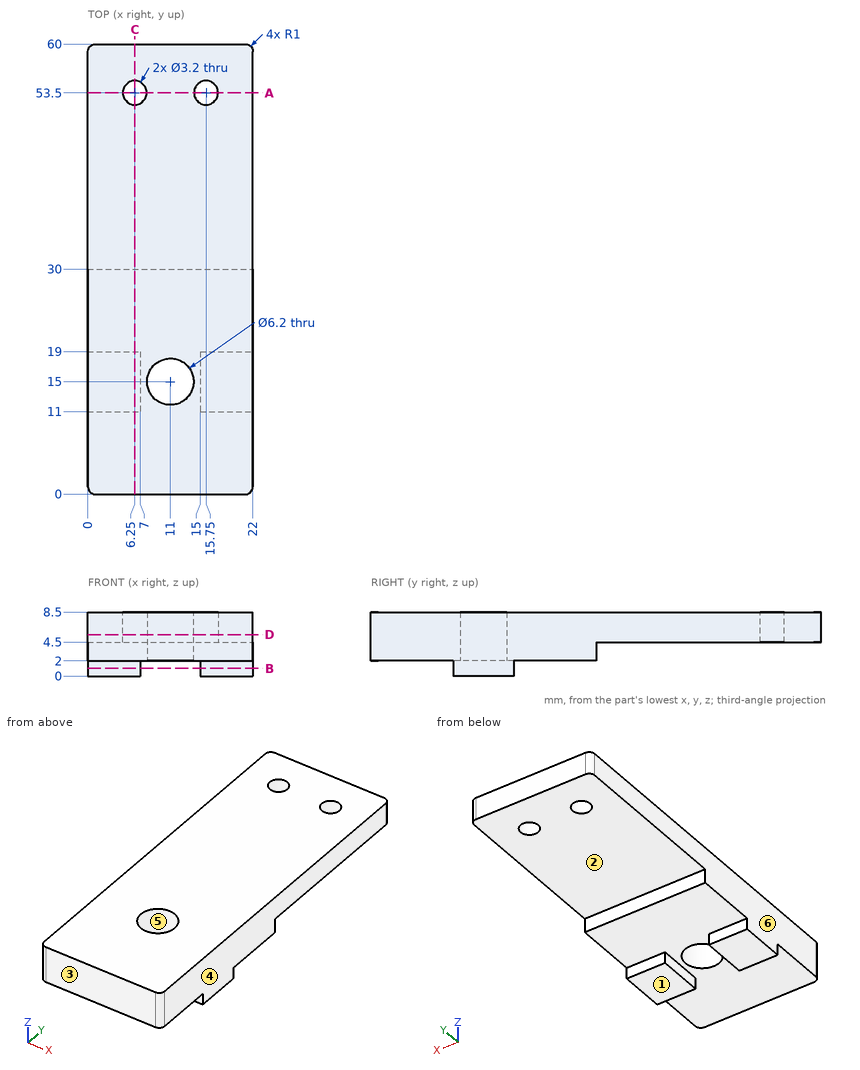
Source: three-view drawing plus pictorial views. Frame: mm from the lowest corner of the part. A direction names the side the tool comes from. Coordinates: 2 decimals unless noted, no trailing zeros. Write each loop counter-clockwise with the first axis right and the second up, starting at its lowest first coordinate (ties: lowest second). Pieces come first, ordered by that corner, then holes. Notation, with made-up numbers: (26, 61) -> (54, 61) arc R27 ccw to (54, 89) -> close; hole circle Ø11 at (62, 26). An arc over 180 degrees is marked (long way). Write each question's results on one line, items separated by ' | '.
Item 1: Set-up query: the marked faces 1 and 2. Return all of +Z, -Z, +X, -X, +Y, -Y with unobstructed straight access to the full face (end or side cutting, diameter ignored); none if empty.
Conclusion:
face 1: -Z, +X, -X, +Y, -Y | face 2: -Z, +X, -X, +Y
Item 2: Section query A-A on y = 53.5. Return loops of the section in (x, z).
Conclusion:
outline: (0, 4.5) -> (4.65, 4.5) -> (4.65, 8.5) -> (0, 8.5) -> close; (7.85, 4.5) -> (14.15, 4.5) -> (14.15, 8.5) -> (7.85, 8.5) -> close; (17.35, 4.5) -> (22, 4.5) -> (22, 8.5) -> (17.35, 8.5) -> close
Item 3: Pin query (flat end, axial travel): pin 1 Ø0.6 at (x, z) = (18, 1) entering from +Y; pin 2 Ø5 at (x, y) = (18, 40) entering from -Z; pin 3 Ø5 at (x, y) = (18, 25.5) entering from -Z; pin 4 Ø2.5 at (x, y) = (15.75, 53.5) entering from +Z. Return the tip coordinate at first contact, or that it passes through.
Conclusion:
pin 1: stops at y = 19 | pin 2: stops at z = 4.5 | pin 3: stops at z = 2 | pin 4: passes through
Item 4: Mould query, pull axis X, two halves, no side actions, for the marked faces 3, 4, 5 and 6. Classes: +X half, -X half, draft (parallel to the pull), parting line (faces both ways), or undercut.
Conclusion:
face 3: draft | face 4: +X half | face 5: undercut | face 6: -X half
Item 5: Material intervals for probe 1 along X at (y, z) = (15, 6.75); probe 2 along Y at (x, z) = (6.25, 5.95); probe 3 along Z at (x, y) = (18.75, 7), sorted ascending.
Conclusion:
probe 1: x = 0 to 7.9, 14.1 to 22 | probe 2: y = 0 to 51.9, 55.1 to 60 | probe 3: z = 2 to 8.5
Item 6: Section query B-B on z = 1. Return loops of the section in (x, y).
Conclusion:
outline: (0, 11) -> (7, 11) -> (7, 19) -> (0, 19) -> close; (15, 11) -> (22, 11) -> (22, 19) -> (15, 19) -> close
Item 7: Section query D-D on z = 5.5. Return loops of the section in (x, y), plus the area to 3 significant figures.
Conclusion:
outline: (0, 1) arc R1 ccw to (1, 0) -> (21, 0) arc R1 ccw to (22, 1) -> (22, 59) arc R1 ccw to (21, 60) -> (1, 60) arc R1 ccw to (0, 59) -> close; hole circle Ø3.2 at (6.25, 53.5); hole circle Ø6.2 at (11, 15); hole circle Ø3.2 at (15.75, 53.5) | area: 1,270 mm^2
Item 8: Section query C-C on x = 6.25. Return loops of the section in (y, z), plus the area to 3 significant figures.
Conclusion:
outline: (0, 2) -> (11, 2) -> (11, 0) -> (19, 0) -> (19, 2) -> (30, 2) -> (30, 4.5) -> (51.9, 4.5) -> (51.9, 8.5) -> (0, 8.5) -> close; (55.1, 4.5) -> (60, 4.5) -> (60, 8.5) -> (55.1, 8.5) -> close | area: 318 mm^2
